The listing builds one solid part. Answer for the finished solid, in the listing's coordinates (mm). Give positions to 0.01 mm unless a question says otherwise; leave off trailing zeros. Loops run counter-clockwise (first coordinate to the right, second up) from the corner with the lowest first, then second, coordinate; pieces in that order, holes last. Notation, with made-up numbers: M 74.25,-18 L 78.25,-18 A9 ccw 78.25,-14 Z; hole C 87,82.25 d11. An arc over 180 degrees is marked long. Use one line per item in the form item = value. Start each with the question number.
1. The part is cut by section A-A (x = 1.3). Write down the section's boundary in (y, z).
2. The part is cut by section D-D (y = -70.5). Write down the section's boundary in (x, z).
3. The part is cut by section C-C (z = -33.5). Write down the section's boundary in (x, y).
4. Straight lines are drawn through the part: line 1 (Z direction, x = 0.3, y = -79); line 2 (Z direction, x = 0.4, y = -79.5); line 3 (Y direction, x = 3.2, z = 80). For each, find the intervals that lie inside material, in ascending order. Write a range as from..to.
5. The part is cut by section B-B (y = -48). Write down the section's boundary in (x, z), and give its area (3 significant figures).
6. Each of these flat-tipped pins is pushed along its axis until it touches: pin 1 Ø1.2 at (x, z) = (2.5, 20) entering from -Y; pin 2 Ø1 at (x, y) = (2, -65) entering from -Z. Where does it stop, or does it pass through?
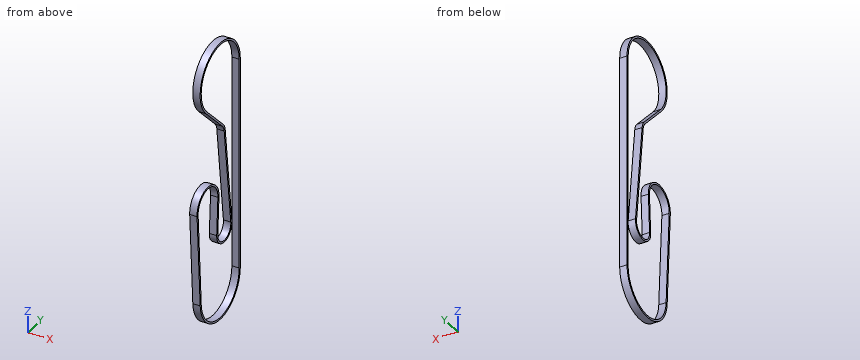
from build123d import *

# Parameters (mm, degrees)
BOSS_EXTRUDE1_DEPTH = 4


with BuildPart() as part:
    # Sketch1 → Boss-Extrude1 (new body)
    with BuildSketch(Plane.YZ):
        with BuildLine():
            Line((-45.297204985, 68.766275416), (-45.297204985, -47.438724583))
            ThreePointArc((-45.297204985, -47.438724583), (-63.559894946, -66.227157099), (-82.858941142, -48.504915228))
            Line((-82.858941142, -48.504915228), (-85.772675501, 2.778943341))
            ThreePointArc((-85.772675501, 2.778943341), (-75.542561207, 13.627257141), (-65.271611457, 2.817597479))
            Line((-65.271611457, 2.817597479), (-66.370650366, -17.905886036))
            ThreePointArc((-66.370650366, -17.905886036), (-60.09842319, -24.321923389), (-54.226508839, -17.537603901))
            Line((-54.226508839, -17.537603901), (-60.400008434, 36.564396099))
            ThreePointArc((-60.400008434, 36.564396099), (-60.963940599, 38.517279926), (-62.138586455, 40.176189762))
            Line((-62.138586455, 40.176189762), (-77.407402535, 55.498956184))
            ThreePointArc((-77.407402535, 55.498956184), (-71.270807609, 86.137850951), (-45.297204985, 68.766275416))
        make_face()
        with BuildLine():
            Line((-81.844577025, -48.447283301), (-84.758311385, 2.836575268))
            ThreePointArc((-84.758311385, 2.836575268), (-75.540645573, 12.611258947), (-66.286185688, 2.871403904))
            Line((-66.286185688, 2.871403904), (-67.385224597, -17.852079611))
            ThreePointArc((-67.385224597, -17.852079611), (-60.067626225, -25.337456524), (-53.217059482, -17.42241712))
            Line((-53.217059482, -17.42241712), (-59.390559076, 36.67958288))
            ThreePointArc((-59.390559076, 36.67958288), (-60.048479935, 38.957947345), (-61.418900101, 40.893342152))
            Line((-61.418900101, 40.893342152), (-76.687716181, 56.216108575))
            ThreePointArc((-76.687716181, 56.216108575), (-70.882829088, 85.198846868), (-46.313204985, 68.766275416))
            Line((-46.313204985, 68.766275416), (-46.313204985, -47.438724583))
            ThreePointArc((-46.313204985, -47.438724583), (-63.588722515, -65.211566152), (-81.844577025, -48.447283301))
        make_face(mode=Mode.SUBTRACT)
    extrude(amount=BOSS_EXTRUDE1_DEPTH)


solid = part.part
Derived:
q1.outline = M -85.77,2.78 L -82.86,-48.5 A18.8 ccw -45.3,-47.44 L -45.3,68.77 A18.8 ccw long -77.41,55.5 L -62.14,40.18 A6.1 cw -60.4,36.56 L -54.23,-17.54 A6.1 cw long -66.37,-17.91 L -65.27,2.82 A10.27 ccw long Z; hole M -84.76,2.84 L -81.84,-48.45 A17.78 ccw -46.31,-47.44 L -46.31,68.77 A17.78 ccw long -76.69,56.22 L -61.42,40.89 A7.11 cw -59.39,36.68 L -53.22,-17.42 A7.11 cw long -67.39,-17.85 L -66.29,2.87 A9.25 ccw long Z
q2.outline = M 0,-65.11 L 4,-65.11 L 4,-64.02 L 0,-64.02 Z; M 0,11.13 L 4,11.13 L 4,12.31 L 0,12.31 Z; M 0,48.57 L 4,48.57 L 4,50.01 L 0,50.01 Z; M 0,85.35 L 4,85.35 L 4,86.44 L 0,86.44 Z
q3.outline = M 0,-83.71 L 4,-83.71 L 4,-82.69 L 0,-82.69 Z; M 0,-46.31 L 4,-46.31 L 4,-45.3 L 0,-45.3 Z
q4.line_1 = -58.89..-57.13, 11.93..13.02, 57.32..59.08, 78.46..80.22
q4.line_2 = -58.21..-56.31, 11.71..12.83, 58..59.89, 77.64..79.53
q4.line_3 = -79.16..-77.87, -50.31..-49.02
q5.outline = M 0,-57.15 L 4,-57.15 L 4,-55 L 0,-55 Z; M 0,76.33 L 4,76.33 L 4,78.48 L 0,78.48 Z
q5.area = 17.2 mm2
q6.pin_1 = -58.58
q6.pin_2 = -66.23
